Could you check a few things on this model? Use its own coordinates, in mm. A direction names the side the tool comes from. Coordinates: 2 decimals unless noted, no trailing zeros. Loops run counter-clockwise (first coordinate to the right, second up) from the corner with the lowest first, then second, coordinate; pieces in that order, holes last. Notation, with made-up numbers: (24, 89.25) - (65, 89.25) arc R29 cw to (65, 123.25) - close; hole circle Ø11 at (71, 33.25). An arc over 180 degrees is marked (long way). Put each result on its own line as item: value. Start each with the question number.
```python
from build123d import *

# Parameters (mm, degrees)
SKETCH1_W           = 45.72
SKETCH1_H           = 22.606
SKETCH1_R           = 1.397
BOSS_EXTRUDE1_DEPTH = 3.175
SKETCH3_R           = 1.5875
BOSS_EXTRUDE2_DEPTH = 3.175
CUT_EXTRUDE1_DEPTH  = 53.966803682
SKETCH5_R           = 1.397
SKETCH5_W           = 2.54
SKETCH5_H           = 1.524
BOSS_EXTRUDE3_DEPTH = 1.524


with BuildPart() as part:
    # Sketch1 → Boss-Extrude1 (new body)
    with BuildSketch(Plane.XY):
        with Locations((22.86, 11.303)):
            Rectangle(SKETCH1_W, SKETCH1_H)
        with Locations((2.54, 3.81)):
            Circle(SKETCH1_R, mode=Mode.SUBTRACT)
        with Locations((43.18, 20.066)):
            Circle(SKETCH1_R, mode=Mode.SUBTRACT)
    extrude(amount=BOSS_EXTRUDE1_DEPTH)

    # Sketch3 → Boss-Extrude2 (add)
    with BuildSketch(Plane(origin=(0, 0, 0), x_dir=(1, 0, 0), z_dir=(0, 1, 0))):
        with BuildLine():
            Line((0, -3.175), (0, 0))
            Line((0, 0), (45.72, 0))
            Line((45.72, 0), (45.72, -3.175))
            ThreePointArc((45.72, -3.175), (45.302298274, -4.570510672), (44.186574776, -5.507039284))
            Line((44.186574776, -5.507039284), (24.747327705, -13.897573657))
            ThreePointArc((24.747327705, -13.897573657), (22.86, -14.2875), (20.972672295, -13.897573657))
            Line((20.972672295, -13.897573657), (1.533425224, -5.507039284))
            ThreePointArc((1.533425224, -5.507039284), (0.417701726, -4.570510672), (0, -3.175))
        make_face()
        with Locations(Location((22.86, -9.525, 0), (0, 0, 270))):
            Circle(SKETCH3_R, mode=Mode.SUBTRACT)
    extrude(amount=-BOSS_EXTRUDE2_DEPTH)

    # Sketch4 → Cut-Extrude1 (cut, through all)
    with BuildSketch(Plane.XY):
        with BuildLine():
            Line((3.175, 18.161), (3.175, 9.332674986))
            ThreePointArc((3.175, 9.332674986), (3.410870982, 8.595465942), (4.030869565, 8.132093467))
            ThreePointArc((4.030869565, 8.132093467), (6.112895277, 6.662648479), (7.084911244, 4.306956522))
            ThreePointArc((7.084911244, 4.306956522), (7.499570341, 3.499427365), (8.34738659, 3.175))
            Line((8.34738659, 3.175), (41.275, 3.175))
            ThreePointArc((41.275, 3.175), (42.173025612, 3.546974388), (42.545, 4.445))
            Line((42.545, 4.445), (42.545, 14.543325014))
            ThreePointArc((42.545, 14.543325014), (42.309129018, 15.280534058), (41.689130435, 15.743906533))
            ThreePointArc((41.689130435, 15.743906533), (39.947107796, 16.833107796), (38.857906533, 18.575130435))
            ThreePointArc((38.857906533, 18.575130435), (38.394534058, 19.195129018), (37.657325014, 19.431))
            Line((37.657325014, 19.431), (4.445, 19.431))
            ThreePointArc((4.445, 19.431), (3.546974388, 19.059025612), (3.175, 18.161))
        make_face()
    extrude(amount=CUT_EXTRUDE1_DEPTH, mode=Mode.SUBTRACT)

    # Sketch5 → Boss-Extrude3 (add)
    # profile 1 of 4: a face of its own
    with BuildSketch(Plane.XY.offset(3.175)):
        with BuildLine():
            Line((2.54, 6.6294), (0, 6.6294))
            Line((0, 6.6294), (0, 0))
            Line((0, 0), (5.3594, 0))
            Line((5.3594, 0), (5.3594, 3.81))
            ThreePointArc((5.3594, 3.81), (4.533616859, 5.803616859), (2.54, 6.6294))
        make_face()
        with Locations((2.54, 3.81)):
            Circle(SKETCH5_R, mode=Mode.SUBTRACT)
    # profile 2 of 4: a face of its own
    with BuildSketch(Plane.XY.offset(3.175)):
        with BuildLine():
            Line((40.259, 20.066), (40.259, 22.606))
            Line((40.259, 22.606), (45.72, 22.606))
            Line((45.72, 22.606), (45.72, 17.145))
            Line((45.72, 17.145), (43.18, 17.145))
            ThreePointArc((43.18, 17.145), (41.114541092, 18.000541092), (40.259, 20.066))
        make_face()
        with Locations((43.18, 20.066)):
            Circle(SKETCH5_R, mode=Mode.SUBTRACT)
    # profile 3 of 4: a face of its own
    with BuildSketch(Plane.XY.offset(3.175)):
        with Locations((1.27, 21.844)):
            Rectangle(SKETCH5_W, SKETCH5_H)
    # profile 4 of 4: a face of its own
    with BuildSketch(Plane.XY.offset(3.175)):
        with Locations((44.45, 0.762)):
            Rectangle(SKETCH5_W, SKETCH5_H)
    extrude(amount=BOSS_EXTRUDE3_DEPTH)


solid = part.part
```
(1) I want a section at A-A on x = 22.86. List the corners of the cut face in (y, z) for me (1 decimal), and give its area (3 significant figures).
(2) If we mould it in two halves opening along Y, with no side actions, what happens to faces 4 (the flat face through (11.39, -1.57, 9.76)), 5 (the cylindrical face through (44.47, 19.53, 2.32)), 6 (the cylindrical face through (4.555, 5.782, 3.926))? For each: pulls with the +Y half, pulls with the -Y half, needs draft (parallel to the pull), parting line crosses it, or undercut.
(3) For pin 1 Ø1.2 at (x, y) = (1, 21.5) entering from +Z; pin 2 Ø1.7 at (x, y) = (43.18, 20.066) entering from +Z; pin 3 Ø1.5 at (x, y) = (12.5, 0) entering from +Z; pin 4 Ø10 at (x, y) = (13.5, 16.5) entering from +Z (3 decimals), each with a flat end and sliding along its axis, tell me the tip position at first contact or that it passes through.
(4) Which directions (+Z, -Z, +X, -X, +Y, -Y) give clear straight access to the entire face, cutting with the end or side of a thin tool? Please do faces 1 (the cylindrical face through (45.314, -1.565, 4.553)), 2 (the cylindrical face through (0.43, -1.57, 4.59)), 3 (the cylindrical face through (39.97, 16.81, 1.57)).
(5) I need wall thicknesses on L1, parallel to Y at x = 10.5, z = 1.75 (3 decimals); L2, parallel to Y at x = 25, z = 9 (3 decimals); L3, parallel to Z at x = 2, y = 19.5 (3 decimals). Which ranges of each line are inside material? Lowest first, please. Write a range as [from, to].
(6) I want a section at B-B on z = 8.5. List the corners of the cut face in (x, y) for me (3 decimals), and give its area (3 significant figures).
(7) I want a section at C-C on x = 18. List the corners of the cut face in (y, z) for me (3 decimals), and give its area (3 significant figures).
(8) I want a section at D-D on z = 13. List the corners of the cut face in (x, y) for me (3 decimals), and give its area (3 significant figures).
Answer sheet:
1. outline: (-3.2, 0) - (3.2, 0) - (3.2, 3.2) - (0, 3.2) - (0, 7.9) - (-3.2, 7.9) - close; (-3.2, 11.1) - (0, 11.1) - (0, 14.3) - (-3.2, 14.3) - close; (19.4, 0) - (22.6, 0) - (22.6, 3.2) - (19.4, 3.2) - close
1. area: 55.4 mm^2
2. face 4: needs draft
2. face 5: undercut
2. face 6: pulls with the +Y half
3. pin 1: stops at z = 4.7
3. pin 2: passes through
3. pin 3: stops at z = 10.56
3. pin 4: stops at z = 3.175
4. face 1: +Z, +X, -Y
4. face 2: +Z, -X, -Y
4. face 3: +Z, -Z
5. L1: y = [-3.175, 3.175], [19.431, 22.606]
5. L2: y = [-3.175, 0]
5. L3: z = [0, 3.175]
6. outline: (8.468, -3.175) - (21.648, -3.175) - (21.648, 0) - (8.468, 0) - close; (24.072, -3.175) - (37.252, -3.175) - (37.252, 0) - (24.072, 0) - close
6. area: 83.7 mm^2
7. outline: (-3.175, 0) - (3.175, 0) - (3.175, 3.175) - (0, 3.175) - (0, 12.614) - (-3.175, 12.614) - close; (19.431, 0) - (22.606, 0) - (22.606, 3.175) - (19.431, 3.175) - close
7. area: 60.2 mm^2
8. outline: (18.893, -3.175) - (26.827, -3.175) - (26.827, 0) - (18.893, 0) - close
8. area: 25.2 mm^2
